Verification items for the finished model (mm, model axes). A direction names the side the tool comes from. Round coordinates to 2 decimals unless told otherwise and drop trailing zeros. Order: outer loops, then holes, each group sorted by start corner. A loop starts at its lowest first (then second) coordinate and runs counter-clockwise, first axis right, second up. Notation, with made-up numbers: (5.25, 48.25) -> (21.25, 48.25) arc R30 ccw to (21.25, 80.25) -> close; hole circle Ø10 at (-3.75, -7.75). An arc over 180 degrees is marked (long way). Put each result on its own line as item: value.
Autodesk Inventor part; units mm, degrees
ref_plane "YZ Plane" through (0, 0, 0) normal (1, 0, 0) x (0, 1, 0)
ref_plane "XZ Plane" through (0, 0, 0) normal (0, 1, 0) x (-1, 0, 0)
ref_plane "XY Plane" through (0, 0, 0) normal (0, 0, 1) x (1, 0, 0)
sketch "スケッチ1" plane through (0, 0, 0) normal (0, 0, 1) x (1, 0, 0)
  line L0 (0, 0) -> (0, 17.65)
  line L1 (0, 17.65) -> (28, 17.65)
  line L2 (28, 17.65) -> (28, 30.15)
  line L3 (28, 30.15) -> (58, 30.15)
  line L4 (58, 30.15) -> (58, 0)
  line L5 (58, 0) -> (60, 0)
  line L6 (60, 0) -> (60, 32.15)
  line L7 (60, 32.15) -> (28, 32.15)
  line L8 (28, 32.15) -> (26, 32.15)
  line L9 (26, 32.15) -> (26, 19.65)
  line L10 (26, 19.65) -> (-2, 19.65)
  line L11 (-2, 19.65) -> (-2, 0)
  line L12 (-2, 0) -> (0, 0)
  dimension "d0" = 17.65
  dimension "d1" = 28
  dimension "d2" = 12.5
  dimension "d3" = 30
  dimension "d4" = 2
  dimension "d5" = 32.15
  dimension "d6" = 32
  dimension "d7" = 2
  dimension "d8" = 12.5
  dimension "d9" = 28
extrude "押し出し1" add sketch "スケッチ1" along normal blind 14
sketch "スケッチ2" plane through (60, 0, 0) normal (1, 0, 0) x (0, 0, -1)
  line L0 (0, 0) -> (-14, 0)
  line L1 (-14, 0) -> (0, 0)
  line L2 (0, 0) -> (0, 2)
  line L3 (0, 2) -> (-14, 2)
  line L4 (-14, 2) -> (-14, 0)
  dimension "d12" = 14
  dimension "d13" = 2
extrude "押し出し2" add sketch "スケッチ2" along normal blind 7
sketch "スケッチ4" plane through (0, 0, 14) normal (0, 0, 1) x (1, 0, 0)
  line L0 (60, 32.15) -> (60, 24.15)
  line L1 (60, 24.15) -> (61.6, 24.15)
  arc A0 (61.6, 20.4) -> (61.6, 27.9) centre (61.6, 24.15) ccw
  line L2 (61.6, 24.15) -> (61.6, 20.4) construction
  line L3 (61.6, 24.15) -> (61.6, 27.9) construction
  line L4 (61.6, 27.9) -> (60, 27.9)
  line L5 (61.6, 20.4) -> (60, 20.4)
  line L6 (60, 2) -> (60, 32.15)
  line L7 (60, 27.9) -> (60, 20.4)
  point P0 (0, 0)
  dimension "d47" = 8
  dimension "d48" = 1.6
  dimension "d49" = 3.75
  dimension "d50" = 180
extrude "押し出し4" add sketch "スケッチ4" against normal blind 14
hole "穴3" at (61.6, 24.15, 14) direction (0, 0, -1) diameter 3.75 end through all
sketch "スケッチ7" plane through (0, 0, 14) normal (0, 0, 1) x (1, 0, 0)
  line L0 (60, 32.15) -> (26, 32.15)
  line L1 (26, 32.15) -> (26, 24.15)
  line L2 (26, 24.15) -> (24.4, 24.15)
  arc A0 (24.4, 27.9) -> (24.4, 20.4) centre (24.4, 24.15) ccw
  line L3 (24.4, 27.9) -> (26, 27.9)
  line L4 (24.4, 20.4) -> (26, 20.4)
  line L5 (26, 20.4) -> (26, 27.9)
  line L6 (26, 32.15) -> (26, 19.65)
  circle A1 centre (24.4, 24.15) radius 1.875
  point P0 (0, 0)
  dimension "d60" = 8
  dimension "d61" = 1.6
  dimension "d62" = 3.75
  dimension "d63" = 3.75
extrude "押し出し6" add sketch "スケッチ7" against normal blind 14 contours L1 A1 L5 L4 A0 L3 | L1 L5 A1 picked at (23.6929, 24.15)
hole "穴4" at (24.4, 24.15, 14) direction (0, 0, -1) diameter 3.75 end through all
sketch "スケッチ10" plane through (0, 17.65, 0) normal (0, -1, 0) x (1, 0, 0)
  line L0 (28, 14) -> (58, 14)
  line L1 (0, 0) -> (28, 0)
  line L2 (28, 0) -> (28, 14)
  line L3 (28, 14) -> (0, 14)
  line L4 (0, 14) -> (0, 0)
extrude "押し出し7" cut sketch "スケッチ10" against normal blind 0.6
sketch "スケッチ11" plane through (0, 0, 0) normal (0, -1, 0) x (1, 0, 0)
  line L0 (-2, 14) -> (0, 14)
  line L1 (60, 0) -> (67, 0)
  line L2 (-9, 14) -> (67, 14)
  line L3 (67, 14) -> (67, 0)
  line L4 (67, 0) -> (-9, 0)
  line L5 (-9, 0) -> (-9, 14)
  point P0 (0, 0)
extrude "押し出し8" cut sketch "スケッチ11" against normal blind 0.6
sketch "スケッチ12" plane through (0, 0, 14) normal (0, 0, 1) x (1, 0, 0)
  line L0 (-2, 19.65) -> (-2, 0.6)
  line L1 (-2, 19.65) -> (4, 19.65)
  line L2 (26, 19.65) -> (-2, 19.65)
  line L3 (4, 19.65) -> (4, 18.25)
  line L4 (0, 18.25) -> (28, 18.25)
  line L5 (4, 18.25) -> (0.2844, 14.5344)
  line L6 (4, 18.25) -> (9.2547, 18.25) construction
  line L7 (0.2844, 14.5344) -> (0, 14.25)
  line L8 (0, 0.6) -> (0, 18.25)
  line L9 (0, 14.25) -> (-2, 14.25)
  line L10 (-2, 14.25) -> (-2, 19.65)
  point P0 (0, 0)
  point P1 (-2, 2)
  dimension "d79" = 6
  dimension "d80" = 135
extrude "押し出し9" add sketch "スケッチ12" along normal blind 2
sketch "スケッチ15" plane through (0, 0, 0) normal (0, 0, -1) x (-1, 0, 0)
  line L0 (0, 0.6) -> (0, 18.25)
  line L1 (0, 18.25) -> (-14, 18.25)
  line L2 (-14, 18.25) -> (-14, 0.6)
  line L3 (-14, 0.6) -> (0, 0.6)
  line L4 (0, 0.6) -> (0, 18.25)
  point P0 (0, 0)
  dimension "d88" = 14
extrude "押し出し11" add sketch "スケッチ15" against normal blind 1.4
sketch "スケッチ17" plane through (67, 0, 0) normal (1, 0, 0) x (0, 0, -1)
  line L0 (0, 0.6) -> (-14, 0.6)
  line L1 (0, 0.6) -> (-14, 0.6)
  line L2 (-14, 0.6) -> (-14, 9.5309)
  line L3 (-14, 9.5309) -> (0, 9.5309)
  line L4 (0, 9.5309) -> (0, 0.6)
  point P0 (0, 0)
extrude "押し出し13" cut sketch "スケッチ17" against normal blind 3
ref_plane "作業平面1" through (-9, 0, 0) normal (-1, 0, 0) x (0, 0, 1)
sketch "スケッチ18" plane through (-9, 0, 0) normal (-1, 0, 0) x (0, 0, 1)
  line L0 (0, 0.6) -> (14, 0.6)
  line L1 (0, 0.6) -> (14, 0.6)
  line L2 (14, 0.6) -> (14, 6.5)
  line L3 (14, 6.5) -> (0, 6.5)
  line L4 (0, 6.5) -> (0, 0.6)
  point P0 (0, 0)
extrude "押し出し14" cut sketch "スケッチ18" against normal blind 3
hole "穴6" at (62, 2, 7) direction (0, -1, 0) diameter 2.4 end through all
sketch "スケッチ19" plane through (0, 0.6, 0) normal (0, -1, 0) x (1, 0, 0)
  line L0 (14, 1.4) -> (14, 0)
  line L1 (14, 0) -> (-2, 0)
  line L2 (-2, 0) -> (-2, -5)
  line L3 (-2, -5) -> (14, -5)
  line L4 (14, -5) -> (14, 0)
  point P0 (0, 0)
  dimension "d115" = 5
extrude "押し出し15" add sketch "スケッチ19" against normal blind 1.4
hole "穴7" at (5, 2, -2.5) direction (0, -1, 0) diameter 2.4 end through all
properties part number "センサ冶具2個積み左"
Item 1: Material ranges on line 1 along X through (y, z) = (24.15, 3) (3 decimals); line 2 along Y through (x, z) = (61.6, 8.25) (3 decimals); line 3 along Z through (x, y) = (5, 1), recorded low to high.
Geometry check:
line 1: 20.65 to 22.525, 26.275 to 28, 58 to 59.725, 63.475 to 65.35
line 2: 0.6 to 2, 20.4 to 22.275, 26.025 to 27.9
line 3: -5 to -3.7, -1.3 to 1.4
Item 2: Sectioned sample at C-C, the plane z = -2.5. Record the boundary of the cut face in (x, y).
Geometry check:
outline: (-2, 0.6) -> (3.8, 0.6) -> (3.8, 2) -> (-2, 2) -> close; (6.2, 0.6) -> (14, 0.6) -> (14, 2) -> (6.2, 2) -> close
Item 3: Depth check by flat-ended pin: pin 1 Ø5 at (y, z) = (7, -2) entering from +X; pin 2 Ø1.2 at (x, y) = (2, 17) entering from -Z; pin 3 Ø5 at (x, y) = (17, 10) entering from -Z; pin 4 Ø2.5 at (x, z) = (2.5, -2) entering from +Y. Enter the tip coordinate at first touch or a pass-through.
Geometry check:
pin 1: x = 60
pin 2: z = 0
pin 3: through
pin 4: y = 2
Item 4: Sectioned sample at D-D, the plane y = 24.15. Record the boundary of the cut face in (x, z) (3 decimals).
Geometry check:
outline: (20.65, 0) -> (22.525, 0) -> (22.525, 14) -> (20.65, 14) -> close; (26.275, 0) -> (28, 0) -> (28, 14) -> (26.275, 14) -> close; (58, 0) -> (59.725, 0) -> (59.725, 14) -> (58, 14) -> close; (63.475, 0) -> (65.35, 0) -> (65.35, 14) -> (63.475, 14) -> close
Item 5: Sectioned sample at A-A, the plane z = 7. Record the boundary of the cut face in (x, y) (3 decimals).
Geometry check:
outline: (-2, 0.6) -> (0, 0.6) -> (0, 18.25) -> (28, 18.25) -> (28, 30.15) -> (58, 30.15) -> (58, 0.6) -> (60.8, 0.6) -> (60.8, 2) -> (60, 2) -> (60, 20.4) -> (61.6, 20.4) arc R3.75 ccw to (61.6, 27.9) -> (60, 27.9) -> (60, 32.15) -> (26, 32.15) -> (26, 27.9) -> (24.4, 27.9) arc R3.75 ccw to (24.4, 20.4) -> (26, 20.4) -> (26, 19.65) -> (-2, 19.65) -> close; (63.2, 0.6) -> (64, 0.6) -> (64, 2) -> (63.2, 2) -> close; hole circle Ø3.75 at (24.4, 24.15); hole circle Ø3.75 at (61.6, 24.15)
Item 6: Sectioned sample at B-B, the plane y = 17. Record the boundary of the cut face in (x, z), then the cut area to 3 significant figures.
Geometry check:
outline: (-2, 0) -> (14, 0) -> (14, 1.4) -> (0, 1.4) -> (0, 14) -> (2.75, 14) -> (2.75, 16) -> (-2, 16) -> close; (58, 0) -> (60, 0) -> (60, 14) -> (58, 14) -> close
area: 85.1 mm2
Item 7: Tool access check on faces 1 (the face through (25, 27.9, 7)), 2 (the face through (25, 20.4, 7)), 3 (the face through (60.81, 1.29, 6.84)), 4 (the face through (28, 24, 7)), 5 (the face through (60, 30, 7)). Record the directions out of +Z, -Z, +X, -X, +Y, -Y that give a thin tool (end or side, any length) a straight path to the whole face; none if there is none.
Geometry check:
face 1: +Z, -Z, -X, +Y
face 2: +Z, -Z, -X
face 3: -Y
face 4: +Z, -Z, -Y
face 5: +Z, -Z, +X, +Y
Item 8: Release check for a two-part mould opening along X. For faces 6 (the face through (43, 32.15, 7)), 7 (the face through (4, 19, 15)), 8 (the face through (7, 10, 1.4)) record: pulls with the +X half, pulls with the -X half, needs draft (parallel to the pull), parting line crosses it, or undercut.
Geometry check:
face 6: needs draft
face 7: pulls with the +X half
face 8: undercut
